```python
from build123d import *

# Parameters (mm, degrees)
SCHIZZO1_R                   = 9
SCHIZZO1_R_2                 = 3
ESTRUSIONE_ESTRUSIONE1_DEPTH = 7
TAGLIO_ESTRUSIONE1_START     = -4
TAGLIO_ESTRUSIONE1_DEPTH     = 4
TAGLIO_ESTRUSIONE2_DEPTH     = 1
RIPETIZIONECIRCOLARE1_COUNT  = 4
ESTRUSIONE_ESTRUSIONE2_DEPTH = 1
ESTRUSIONE_ESTRUSIONE3_DEPTH = 2
SCHIZZO7_R                   = 1.75
ESTRUSIONE_ESTRUSIONE4_DEPTH = 15
RACCORDO1_R                  = 0.5


with BuildPart() as part:
    # Schizzo1 → Estrusione-Estrusione1 (new body)
    with BuildSketch(Plane(origin=(0, 0, 0), x_dir=(1, 0, 0), z_dir=(0, 1, 0))):
        with Locations(Location((0, 0, 0), (0, 0, 270))):
            Circle(SCHIZZO1_R)
        with Locations(Location((0, 0, 0), (0, 0, 270))):
            Circle(SCHIZZO1_R_2, mode=Mode.SUBTRACT)
    extrude(amount=ESTRUSIONE_ESTRUSIONE1_DEPTH)

    # Schizzo3 → Taglio-Estrusione1 (cut)
    with BuildSketch(Plane(origin=(0, 7, 0), x_dir=(1, 0, 0), z_dir=(0, 1, 0)).offset(TAGLIO_ESTRUSIONE1_START)):
        with BuildLine():
            Line((7.193747285, 3.5), (8.092965696, 3.9375))
            ThreePointArc((8.092965696, 3.9375), (-9, 0), (8.092965696, -3.9375))
            Line((8.092965696, -3.9375), (7.193747285, -3.5))
            ThreePointArc((7.193747285, -3.5), (8, 0), (7.193747285, 3.5))
        make_face()
    extrude(amount=TAGLIO_ESTRUSIONE1_DEPTH, mode=Mode.SUBTRACT)

    # Schizzo4 → Taglio-Estrusione2 (cut)
    with BuildSketch(Plane(origin=(0, 3, 0), x_dir=(1, 0, 0), z_dir=(0, 1, 0))):
        with BuildLine():
            Line((-0.5, 4.974937186), (-0.5, 7.483314774))
            ThreePointArc((-0.5, 7.483314774), (-5.303300859, 5.303300859), (-7.483314774, 0.5))
            Line((-7.483314774, 0.5), (-4.974937186, 0.5))
            ThreePointArc((-4.974937186, 0.5), (-3.535533906, 3.535533906), (-0.5, 4.974937186))
        make_face()
    taglio_estrusione2 = extrude(amount=-TAGLIO_ESTRUSIONE2_DEPTH, mode=Mode.SUBTRACT)

    # RipetizioneCircolare1: Taglio-Estrusione2 ×4 about axis
    ripetizionecircolare1_axis = Axis((0, 0, 0), (0, 1, 0))
    for i in range(1, RIPETIZIONECIRCOLARE1_COUNT):
        add(taglio_estrusione2.rotate(ripetizionecircolare1_axis, i * 360 / RIPETIZIONECIRCOLARE1_COUNT), mode=Mode.SUBTRACT)

    # Schizzo5 → Estrusione-Estrusione2 (add)
    with BuildSketch(Plane(origin=(0, 0, 0), x_dir=(1, 0, 0), z_dir=(0, 1, 0))):
        with BuildLine():
            Line((0, 9), (0, 12.5))
            ThreePointArc((0, 12.5), (-2.091650066, 12.323757544), (-4.124318125, 11.8))
            Line((-4.124318125, 11.8), (-11.456439237, 5))
            ThreePointArc((-11.456439237, 5), (-12.5, 0), (-11.456439237, -5))
            Line((-11.456439237, -5), (-4.124318125, -11.8))
            ThreePointArc((-4.124318125, -11.8), (-2.091650066, -12.323757544), (0, -12.5))
            Line((0, -12.5), (0, -9))
            ThreePointArc((0, -9), (-9, 0), (0, 9))
        make_face()
    extrude(amount=ESTRUSIONE_ESTRUSIONE2_DEPTH)

    # Schizzo6 → Estrusione-Estrusione3 (add)
    with BuildSketch(Plane(origin=(0, 1, 0), x_dir=(1, 0, 0), z_dir=(0, 1, 0))):
        with BuildLine():
            Line((-8.986100378, 0.5), (-11.286100378, 0.5))
            ThreePointArc((-11.286100378, 0.5), (-11.427521734, 0.441421356), (-11.486100378, 0.3))
            Line((-11.486100378, 0.3), (-11.486100378, -0.3))
            ThreePointArc((-11.486100378, -0.3), (-11.427521734, -0.441421356), (-11.286100378, -0.5))
            Line((-11.286100378, -0.5), (-8.986100378, -0.5))
            ThreePointArc((-8.986100378, -0.5), (-9, 0), (-8.986100378, 0.5))
        make_face()
    extrude(amount=ESTRUSIONE_ESTRUSIONE3_DEPTH)

    # Schizzo7 → Estrusione-Estrusione4 (add)
    with BuildSketch(Plane.XZ):
        with Locations(Location((-9.287087811, 2, 0), (0, 0, 90))):
            Circle(SCHIZZO7_R)
    extrude(amount=ESTRUSIONE_ESTRUSIONE4_DEPTH)

    # Raccordo1
    raccordo1_edges = [part.edges().sort_by_distance(p)[0] for p in [
        (-9.287087811, -15, 0.25),
    ]]
    fillet(raccordo1_edges, radius=RACCORDO1_R)


solid = part.part
```
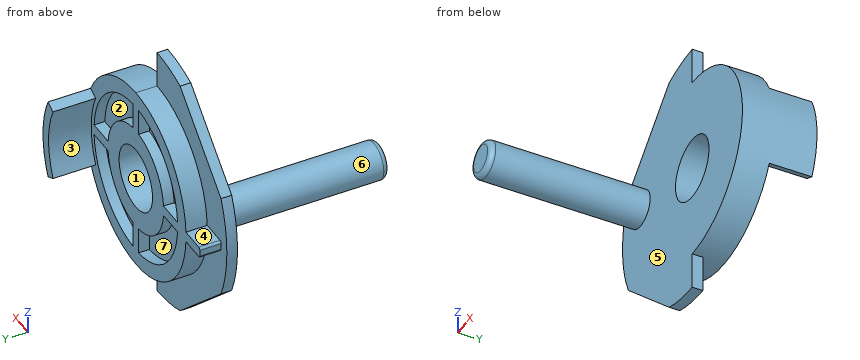
Work out the finished part from the listing and answer in its coordinate system (mm). Face numbers are marked on the shaded views. A direction names the side the tool comes from. Give positions to 0.01 mm unless a question says otherwise; leave off trailing zeros. Write each loop counter-clockwise with the first axis right and the second up, starting at its lowest first coordinate (ties: lowest second). Pieces come first, ordered by that corner, then holes.
(1) Flat-ended cylindrical pins translate along their axes: pin 1 Ø1.1 at (x, y) = (6, 2.5) entering from +Z; pin 2 Ø1.5 at (x, y) = (-7, -3.5) entering from +Z; pin 3 Ø10 at (x, z) = (-7, 1.5) entering from +Y. Find the tip coordinate at first contact, or state that the pin passes through.
Final values:
pin 1: stops at z = 7.16
pin 2: stops at z = 2.84
pin 3: stops at y = 3
(2) The part is cut by section A-A on z = -1.25. Write down the section's boundary in (x, y).
Final values:
outline: (-12.44, 0) - (-2.73, 0) - (-2.73, 3) - (-4.84, 3) - (-4.84, 2) - (-7.4, 2) - (-7.4, 3) - (-8.91, 3) - (-8.91, 1) - (-12.44, 1) - close; (2.73, 0) - (8.91, 0) - (8.91, 7) - (7.9, 7) - (7.9, 3) - (7.4, 3) - (7.4, 2) - (4.84, 2) - (4.84, 3) - (2.73, 3) - close
(3) The part is cut by section D-D on x = -6.5. Write down the section's boundary in (y, z), plus the area to 3 significant figures.
Final values:
outline: (0, -9.6) - (1, -9.6) - (1, -6.22) - (3, -6.22) - (3, -3.74) - (2, -3.74) - (2, -0.5) - (3, -0.5) - (3, 0.5) - (2, 0.5) - (2, 3.74) - (3, 3.74) - (3, 6.22) - (1, 6.22) - (1, 9.6) - (0, 9.6) - close
area: 37.6 mm2
(4) The part is cut by section C-C on y = 4. Write down the section's boundary in (x, z).
Final values:
outline: (7.19, -3.5) - (8.09, -3.94) arc R9 ccw to (8.09, 3.94) - (7.19, 3.5) arc R8 cw to start
(5) The part is cut by section B-B on x = -1.5. Write down the section's boundary in (y, z), plus the area to 3 significant figures.
Final values:
outline: (0, -12.41) - (1, -12.41) - (1, -8.87) - (3, -8.87) - (3, -7.35) - (2, -7.35) - (2, -4.77) - (3, -4.77) - (3, -2.6) - (0, -2.6) - close; (0, 2.6) - (3, 2.6) - (3, 4.77) - (2, 4.77) - (2, 7.35) - (3, 7.35) - (3, 8.87) - (1, 8.87) - (1, 12.41) - (0, 12.41) - close
area: 39.6 mm2
(6) Which of the six approach directions +Z, -Z, +X, -X, +Y, -Y give full straight-line access (tool end or side, diameter ignored) to the marked faces 1, 2 and 3?
Final values:
face 1: +Y, -Y
face 2: +Y
face 3: -X, +Y
(7) The mould has two halves that part along Z. Classify the marked faces 4, 5, 6 and 7: pulls with the +Z half, pulls with the -Z half, needs draft (parallel to the pull), parting line crosses it, or undercut.
Final values:
face 4: pulls with the +Z half
face 5: needs draft
face 6: parting line crosses it
face 7: undercut
(8) Straight lines are drawn through the part: line 1 (Z direction, x = 0, y = 2.2); line 2 (X direction, y = 1.4, z = 0); line 3 (Y direction, x = 1.25, z = -3.5). For each, find the intervals that lie inside material, in ascending order.
Final values:
line 1: z = -9 to -3, 3 to 9
line 2: x = -11.49 to -3, 3 to 9
line 3: y = 0 to 3
